```python
from build123d import *

# Parameters (mm, degrees)
F0_W     = 44.45
F0_H     = 203.2
F1_DEPTH = 2.54
F2_R     = 5.08
F3_R     = 1.27
F4_DEPTH = 2.54
F5_R     = 1.27
F6_R     = 1.27
F7_DEPTH = 2.54
F8_R     = 1.27


with BuildPart() as f1:
    # F0 (on Right) → F1 (new body)
    with BuildSketch(Plane.YZ):
        with Locations((32.198633, 1.147029)):
            Rectangle(F0_W, F0_H)
    extrude(amount=-F1_DEPTH)

    # F2
    f2_edges = [f1.edges().sort_by_distance(p)[0] for p in [
        (-1.27, 54.423633, 102.747029),
        (-1.27, 9.973633, 102.747029),
        (-1.27, 54.423633, -100.452971),
        (-1.27, 9.973633, -100.452971),
    ]]
    fillet(f2_edges, radius=F2_R)

    # F3 (on face) → F4 (join)
    with BuildSketch(Plane(origin=(-2.54, 0, 0), x_dir=(0, -1, 0), z_dir=(-1, 0, 0))):
        with Locations((-32.198633, 95.127029)):
            Circle(F3_R)
    extrude(amount=F4_DEPTH)

    # F5
    f5_edges = [f1.edges().sort_by_distance(p)[0] for p in [
        (-5.08, 33.468633, 95.127029),
    ]]
    fillet(f5_edges, radius=F5_R)

    # F6 (on face) → F7 (join)
    with BuildSketch(Plane(origin=(-2.54, 0, 0), x_dir=(0, -1, 0), z_dir=(-1, 0, 0))):
        with Locations((-32.198633, -92.832971)):
            Circle(F6_R)
    extrude(amount=F7_DEPTH)

    # F8
    f8_edges = [f1.edges().sort_by_distance(p)[0] for p in [
        (-5.08, 33.468633, -92.832971),
    ]]
    fillet(f8_edges, radius=F8_R)


solid = f1.part
```
The listing builds one solid part. Answer for the finished solid, in the listing's coordinates (mm). Give positions to 0.01 mm unless a question says otherwise; leave off trailing zeros. Write each loop counter-clockwise with the first axis right and the second up, starting at its lowest first coordinate (ties: lowest second). Pieces come first, ordered by that corner, then holes. Notation, with made-up numbers: M -10,39 L 4,39 A12 ccw 4,49 Z; hole C 50,-36 d10. An arc over 180 degrees is marked long. Write each question's results on one line, items separated by ' | '.
Q1. Flat-ended cylindrical pins translate along their axes: P1, Ø22, axis at y = 22, z = -32, coming from the -X side; P2, Ø2, axis at x = -4.5, z = -2.5, coming from the -Y side. Find the tip coordinate at first contact, or state that the pin passes through.
Output values:
P1: x = -2.54 | P2: through
Q2. Section B-B, the plane y = 36.5 is taken. Write down the section's boundary in (x, z).
Output values:
outline: M -2.54,-100.45 L 0,-100.45 L 0,102.75 L -2.54,102.75 Z
Q3. Consider L1, parallel to X at y = 23, z = 76.5; L2, parallel to Z at x = -1.3, y = 52. Determine where each line is inside the solid, lowest interval first. Write a range as from..to.
Output values:
L1: -2.54..0 | L2: -99.7..102
Q4. Section A-A, the plane z = -79 is taken. Write down the section's boundary in (x, y), then the cut area to 3 significant figures.
Output values:
outline: M -2.54,9.97 L 0,9.97 L 0,54.42 L -2.54,54.42 Z | area: 113 mm2
